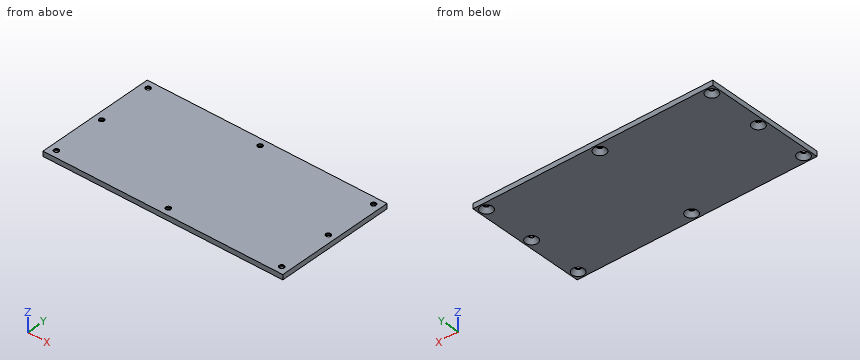
```python
from build123d import *

# Parameters (mm, degrees)
F0_W           = 152.4
F0_H           = 76.2
F1_DEPTH       = 3.175
F3_D           = 3.175
F3_CSINK_D     = 7.62
F3_CSINK_ANGLE = 82


with BuildPart() as f1:
    # F0 (on Top) → F1 (new body)
    with BuildSketch(Plane.XY):
        with Locations((76.2, 38.1)):
            Rectangle(F0_W, F0_H)
    extrude(amount=F1_DEPTH)

    # F3 (through all)
    with Locations(Plane(origin=(0, 0, 0), x_dir=(1, 0, 0), z_dir=(0, 0, -1))):
        with Locations((4.572, -4.572), (4.572, -37.592), (4.572, -71.628), (75.692, -71.628), (147.828, -71.628), (147.828, -38.608), (147.828, -457.2), (75.692, -4.572), (147.763029, -4.572)):
            CounterSinkHole(F3_D / 2, F3_CSINK_D / 2, counter_sink_angle=F3_CSINK_ANGLE)


solid = f1.part
```
Design review of the part built by this model. Coordinates are the model's own, in mm. Coordinates: 2 decimals unless noted, no trailing zeros. One line per item, written item: value. Start each with the question number.
Q1. For probe 1 along X at (y, z) = (6, 1.05); probe 2 along X at (y, z) = (70, 2); probe 3 along X at (y, z) = (38.5, 1.9), list the stretches that pass through material, from the lowest coordinate up.
Q2. Insertion check: pin 1 Ø3 at (x, y) = (4.572, 71.628) entering from -Z; pin 2 Ø4 at (x, y) = (75.692, 4.572) entering from -Z. Each pin has a flat end and moves straight along its axis. Give the tip position at first contact, or say it passes through.
Q3. Take a section at A-A, the plane z = 0.7. Give the number of separate pieces and of enclosed holes in the cut face, then the cut area to 3 significant figures.
Values follow:
1. probe 1: x = 0 to 2.05, 7.09 to 73.17, 78.21 to 145.24, 150.28 to 152.4
1. probe 2: x = 0 to 3.29, 5.85 to 74.41, 76.97 to 146.55, 149.11 to 152.4
1. probe 3: x = 0 to 2.61, 6.53 to 145.67, 149.98 to 152.4
2. pin 1: passes through
2. pin 2: stops at z = 2.08
3. separate pieces: 1
3. enclosed holes: 8
3. area: 11,400 mm2
